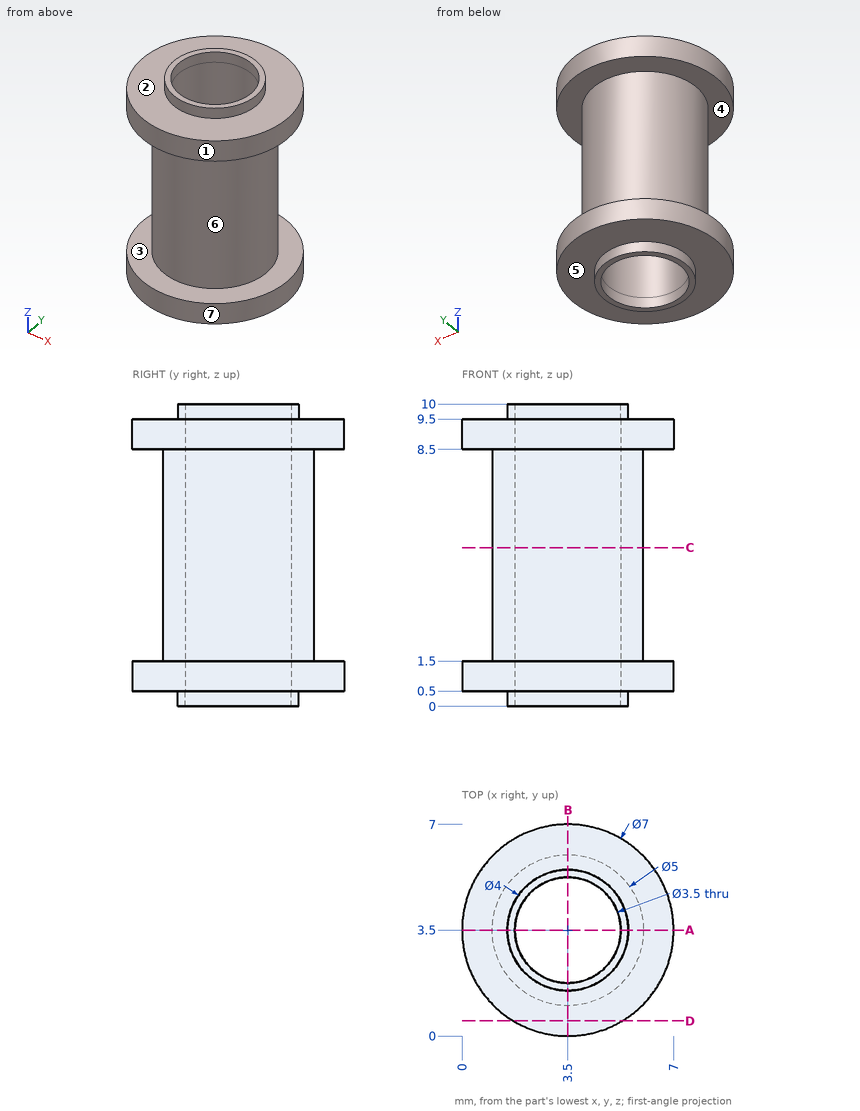
Design review of the part shown in the three views and the two pictorial views. Dimensions are in mm from the part's minimum x, y and z. A direction names the side the tool comes from. Give positions to 0.01 mm unless a question says otherwise; leave off trailing zeros. Write each loop counter-clockwise with the first axis right and the second up, starting at its lowest first coordinate (ties: lowest second). Pieces come first, ordered by that corner, then holes. Notation, with made-up numbers: M 24,17 L 35,17 A31 cw 35,56 Z; hole C 84.25,-14.5 d6. An arc over 180 degrees is marked long. One line per item, written item: value.
1) The part is to be moulded in two halves that separate along Z. For the marked faces 1, 2, 3 and 4, say which applies: +Z half, -Z half, draft (parallel to the pull), parting line (faces both ways), or undercut.
Results are:
face 1: draft
face 2: +Z half
face 3: undercut
face 4: undercut
2) For line 1 (Z direction, x = 6.25, y = 2.25); line 2 (Y direction, x = 3.5, z = 0.45); line 3 (X direction, y = 3.5, z = 4.75), list the stretches that pass through material, from the lowest coordinate up. Write a range as from..to.
Results are:
line 1: z = 0.5..1.5, 8.5..9.5
line 2: y = 1.5..1.75, 5.25..5.5
line 3: x = 1..1.75, 5.25..6
3) For P1, Ø1.5, axis at x = 4.5, z = 4.5, coming from the +Y side; P2, Ø3.5, axis at x = 3, y = 4.5, coming from the -Z side, all flat-tipped, find the tip position at first contact; note any pin that passes through.
Results are:
P1: stops at y = 5.99
P2: stops at z = 0
4) For the marked faces 5, 6 and 7, list the 3-axis set-ups (+Z, -Z, +X, -X, +Y, -Y) from which the entire face can be reached by the end or side of a thin tool; tool diameter is ignored.
Results are:
face 5: -Z
face 6: none
face 7: +Z, -Z
5) Take a section at C-C, the plane z = 5.25. Write out the cut boundary in (x, y), then the cut area to 3 significant figures.
Results are:
outline: C 3.5,3.5 d5; hole C 3.5,3.5 d3.5
area: 10.0 mm²
6) Take a section at D-D, the plane y = 0.5. Write out the cut boundary in (x, z).
Results are:
outline: M 1.7,0.5 L 5.3,0.5 L 5.3,1.5 L 1.7,1.5 Z; M 1.7,8.5 L 5.3,8.5 L 5.3,9.5 L 1.7,9.5 Z
7) Take a section at A-A, the plane y = 3.5. Write out the cut boundary in (x, z), then the cut area to 3 significant figures.
Results are:
outline: M 0,0.5 L 1.5,0.5 L 1.5,0 L 1.75,0 L 1.75,10 L 1.5,10 L 1.5,9.5 L 0,9.5 L 0,8.5 L 1,8.5 L 1,1.5 L 0,1.5 Z; M 5.25,0 L 5.5,0 L 5.5,0.5 L 7,0.5 L 7,1.5 L 6,1.5 L 6,8.5 L 7,8.5 L 7,9.5 L 5.5,9.5 L 5.5,10 L 5.25,10 Z
area: 18.0 mm²
